```python
from build123d import *

# Parameters (mm, degrees)
SKETCH1_W                   = 38.1
SKETCH1_H                   = 38.1
BOSS_EXTRUDE1_DEPTH         = 6.35
SKETCH2_R                   = 9.525
CUT_EXTRUDE1_DEPTH          = 28.679008291
SKETCH3_R                   = 0.635
CUT_EXTRUDE2_DEPTH          = 44.067795393
CIRPATTERN1_COUNT           = 4
SKETCH4_R                   = 0.635
CUT_EXTRUDE3_DEPTH          = 5.08
CIRPATTERN2_COUNT           = 4
TAP_DRILL_FOR_1_4_20_TAP1_D = 5.1054


with BuildPart() as part:
    # Sketch1 → Boss-Extrude1 (new body)
    with BuildSketch(Plane(origin=(0, 0, 0), x_dir=(1, 0, 0), z_dir=(0, 1, 0))):
        Rectangle(SKETCH1_W, SKETCH1_H)
    extrude(amount=BOSS_EXTRUDE1_DEPTH)

    # Sketch2 → Cut-Extrude1 (cut, through all)
    with BuildSketch(Plane.XZ):
        with Locations(Location((0, 0, 0), (0, 0, 270))):
            Circle(SKETCH2_R)
    extrude(amount=-CUT_EXTRUDE1_DEPTH, mode=Mode.SUBTRACT)

    # Sketch3 → Cut-Extrude2 (cut, through all)
    with BuildSketch(Plane.XY.offset(19.05)):
        with Locations((0, 1.524)):
            Circle(SKETCH3_R)
    cut_extrude2 = extrude(amount=-CUT_EXTRUDE2_DEPTH, mode=Mode.SUBTRACT)

    # CirPattern1: Cut-Extrude2 ×4 about axis
    cirpattern1_axis = Axis((0, 6.35, 0), (0, -1, 0))
    for i in range(1, CIRPATTERN1_COUNT):
        add(cut_extrude2.rotate(cirpattern1_axis, i * 360 / CIRPATTERN1_COUNT), mode=Mode.SUBTRACT)

    # Sketch4 → Cut-Extrude3 (cut)
    with BuildSketch(Plane.XY.offset(19.05)):
        with Locations((0, 4.445)):
            Circle(SKETCH4_R)
    cut_extrude3 = extrude(amount=-CUT_EXTRUDE3_DEPTH, mode=Mode.SUBTRACT)

    # CirPattern2: Cut-Extrude3 ×4 about axis
    cirpattern2_axis = Axis((0, 0, 0), (0, 1, 0))
    for i in range(1, CIRPATTERN2_COUNT):
        add(cut_extrude3.rotate(cirpattern2_axis, i * 360 / CIRPATTERN2_COUNT), mode=Mode.SUBTRACT)

    # Tap Drill for 1/4-20 Tap1 (through all)
    with Locations(Plane(origin=(0, 6.35, 0), x_dir=(1, 0, 0), z_dir=(0, 1, 0))):
        with Locations((-13.97, 13.97), (13.97, 13.97), (-13.97, -13.97), (13.97, -13.97)):
            Hole(TAP_DRILL_FOR_1_4_20_TAP1_D / 2)


solid = part.part
```
Geometry: final body of the model. Coordinates: model frame, mm. A direction names the side the tool comes from. Coordinates: 2 decimals unless noted, no trailing zeros. Write each loop counter-clockwise with the first axis right and the second up, starting at its lowest first coordinate (ties: lowest second). Pieces come first, ordered by that corner, then holes. Notation, with made-up numbers: M 44.25,30 L 77.25,30 A18 cw 77.25,65 Z; hole C -9,-20 d4. An arc over 180 degrees is marked long. Answer as CSV lines item,"result". Start each with the question number.
Q1. Reachability of faces 1 (the cylindrical face through (-16.546, 3.825, -0.138)), 2 (the cylindrical face through (16.546, 3.825, 0.138)), 3 (the flat face through (0, 4, 13.97)), 4 (the cylindrical face through (0.138, 3.825, -16.546)) from +Z, -Z, +X, -X, +Y, -Y: full face, straight path, thin tool, end or side. Return the list, or none.
Q2. Cut plane D-D on x = -3. Return the cut outline in (y, z).
Q3. Pin query (flat end, axial travel): P1, Ø4, axis at x = -5, z = -13.5, coming from the -Y side; P2, Ø0.8, axis at x = 0, y = 4.445, coming from the +Z side; P3, Ø1.1, axis at y = 1.524, z = 0, coming from the +X side; P4, Ø0.6, axis at x = 0, y = 4.5, coming from the -Z side. Return the tip coordinate at first contact, or that it passes through.
Q4. Line query: line 1 (Z direction, x = -14, y = 6.25); line 2 (Y direction, x = 15, z = 0). Output: solid intervals per line, ascending. Write a range as from..to.
Q5. Mould query, pull axis Y, two halves, no side actions, for faces 5 (the flat face through (0, 3, -19.05)), 6 (the flat face through (-5, 0, -9)), 7 (the flat face through (-5, 6.35, -9)), 8 (the cylindrical face through (-0.083, 2.154, 14.344)). Classes: released by +Y, released by -Y, zero draft, split by the parting line, or undercut.
Q6. Cut plane A-A on y = 3. Return the cut outline in (x, z) (3 decimals), then the cut area to 3 significant figures.
Q7. Cut plane B-B on z = 15. Return the cut outline in (x, y) (3 decimals).
Q8. Cut plane C-C on x = 13. Return the cut outline in (y, z) (3 decimals).
Findings below:
1,face 1,"-X"
1,face 2,"+X"
1,face 3,"+Z"
1,face 4,"-Z"
2,outline,"M 0,-19.05 L 6.35,-19.05 L 6.35,-9.04 L 0,-9.04 Z; M 0,9.04 L 6.35,9.04 L 6.35,19.05 L 0,19.05 Z"
3,P1,"stops at y = 0"
3,P2,"stops at z = 13.97"
3,P3,"passes through"
3,P4,"stops at z = -13.97"
4,line 1,"z = -19.05..-16.52, -11.42..11.42, 16.52..19.05"
4,line 2,"y = 0..0.89, 2.16..3.81, 5.08..6.35"
5,face 5,"zero draft"
5,face 6,"released by -Y"
5,face 7,"released by +Y"
5,face 8,"undercut"
6,outline,"M -19.05,-19.05 L 19.05,-19.05 L 19.05,19.05 L -19.05,19.05 Z; hole C -13.97,-13.97 d5.105; hole C -13.97,13.97 d5.105; hole C 0,0 d19.05; hole C 13.97,-13.97 d5.105; hole C 13.97,13.97 d5.105"
6,area,"1,080 mm2"
7,outline,"M -19.05,0 L -16.306,0 L -16.306,6.35 L -19.05,6.35 Z; M -11.634,0 L 11.634,0 L 11.634,6.35 L -11.634,6.35 Z; M 16.306,0 L 19.05,0 L 19.05,6.35 L 16.306,6.35 Z; hole C 0,1.524 d1.27; hole C 0,4.445 d1.27"
8,outline,"M 0,-19.05 L 6.35,-19.05 L 6.35,-16.331 L 0,-16.331 Z; M 0,-11.609 L 6.35,-11.609 L 6.35,11.609 L 0,11.609 Z; M 0,16.331 L 6.35,16.331 L 6.35,19.05 L 0,19.05 Z; hole C 1.524,0 d1.27"
